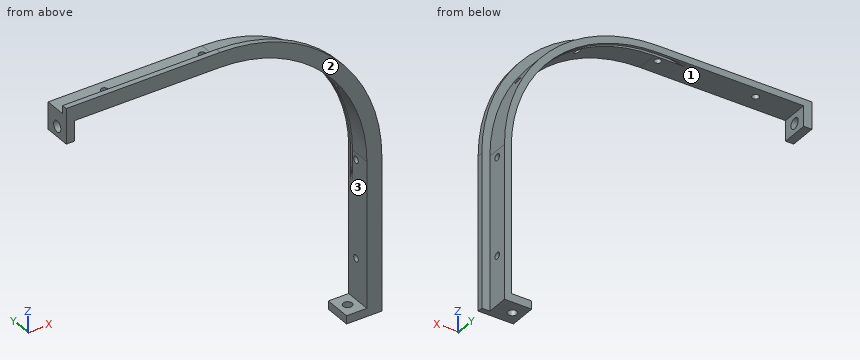
from build123d import *

# Parameters (mm, degrees)
BOSS_EXTRUDE1_DEPTH = 10
CUT_EXTRUDE1_START  = -1
SKETCH2_R           = 55.1
CUT_EXTRUDE1_DEPTH  = 1.1
CUT_EXTRUDE2_DEPTH  = 8
SKETCH4_R           = 2
CUT_EXTRUDE3_DEPTH  = 4
SKETCH5_R           = 1.65
CUT_EXTRUDE4_DEPTH  = 4
SKETCH7_R           = 1.25
CUT_EXTRUDE5_DEPTH  = 114.07
SKETCH9_R           = 1.25
CUT_EXTRUDE6_DEPTH  = 134.776057092


with BuildPart() as part:
    # Sketch1 → Boss-Extrude1 (new body)
    with BuildSketch(Plane(origin=(0, 0, 0), x_dir=(1, 0, 0), z_dir=(0, 1, 0))):
        with BuildLine():
            Line((0, -116.07), (56.57, -116.07))
            ThreePointArc((56.57, -116.07), (98.642853481, -98.642853481), (116.07, -56.57))
            Line((116.07, -56.57), (116.07, 0))
            Line((116.07, 0), (103.07, 0))
            Line((103.07, 0), (103.07, -3))
            Line((103.07, -3), (110.57, -3))
            Line((110.57, -3), (110.57, -56.57))
            ThreePointArc((110.57, -56.57), (94.753766184, -94.753766184), (56.57, -110.57))
            Line((56.57, -110.57), (3, -110.57))
            Line((3, -110.57), (3, -103.07))
            Line((3, -103.07), (0, -103.07))
            Line((0, -103.07), (0, -116.07))
        make_face()
    extrude(amount=BOSS_EXTRUDE1_DEPTH)

    # Sketch2 → Cut-Extrude1 (cut)
    with BuildSketch(Plane(origin=(0, 10, 0), x_dir=(1, 0, 0), z_dir=(0, 1, 0)).offset(CUT_EXTRUDE1_START)):
        with Locations((56.57, -56.57)):
            Circle(SKETCH2_R)
    extrude(amount=-CUT_EXTRUDE1_DEPTH, mode=Mode.SUBTRACT)

    # Sketch3 → Cut-Extrude2 (cut)
    with BuildSketch(Plane(origin=(0, 10, 0), x_dir=(1, 0, 0), z_dir=(0, 1, 0))):
        with BuildLine():
            Line((113.07, -56.57), (113.07, 0))
            Line((113.07, 0), (116.07, 0))
            Line((116.07, 0), (116.07, -56.57))
            ThreePointArc((116.07, -56.57), (98.642853481, -98.642853481), (56.57, -116.07))
            Line((56.57, -116.07), (0, -116.07))
            Line((0, -116.07), (0, -113.07))
            Line((0, -113.07), (56.57, -113.07))
            ThreePointArc((56.57, -113.07), (96.521533137, -96.521533137), (113.07, -56.57))
        make_face()
    extrude(amount=-CUT_EXTRUDE2_DEPTH, mode=Mode.SUBTRACT)

    # Sketch4 → Cut-Extrude3 (cut, through all)
    with BuildSketch(Plane(origin=(3, 0, 0), x_dir=(0, 0, -1), z_dir=(1, 0, 0))):
        with Locations((-106.82, 5)):
            Circle(SKETCH4_R)
    extrude(amount=-CUT_EXTRUDE3_DEPTH, mode=Mode.SUBTRACT)

    # Sketch5 → Cut-Extrude4 (cut, through all)
    with BuildSketch(Plane.XY.offset(3)):
        with Locations((106.82, 5)):
            Circle(SKETCH5_R)
    extrude(amount=-CUT_EXTRUDE4_DEPTH, mode=Mode.SUBTRACT)

    # Sketch7 → Cut-Extrude5 (cut, through all)
    with BuildSketch(Plane.XY.offset(113.07)):
        with Locations((18, 6)):
            Circle(SKETCH7_R)
        with Locations((54, 6)):
            Circle(SKETCH7_R)
    cut_extrude5 = extrude(amount=-CUT_EXTRUDE5_DEPTH, mode=Mode.SUBTRACT)

    # Sketch9 → Cut-Extrude6 (cut, through all)
    with BuildSketch(Plane(origin=(66.888028546, 0, 115.85346386), x_dir=(-0.866025404, 0, 0.5), z_dir=(-0.5, 0, -0.866025404))):
        with Locations((-20.706057092, 6)):
            Circle(SKETCH9_R)
    cut_extrude6 = extrude(amount=CUT_EXTRUDE6_DEPTH, mode=Mode.SUBTRACT)

    # Mirror1: Cut-Extrude5, Cut-Extrude6 across plane
    add(cut_extrude5.mirror(Plane(origin=(0, 0, 0), x_dir=(0.707106781, 0, 0.707106781), z_dir=(-0.707106781, 0, 0.707106781))), mode=Mode.SUBTRACT)
    add(cut_extrude6.mirror(Plane(origin=(0, 0, 0), x_dir=(0.707106781, 0, 0.707106781), z_dir=(-0.707106781, 0, 0.707106781))), mode=Mode.SUBTRACT)


solid = part.part
Geometry: final body of the model. Coordinates: model frame, mm. Face numbers are marked on the shaded views. Round coordinates to 2 decimals unless told otherwise and drop trailing zeros. Loops run counter-clockwise (first coordinate to the right, second up) from the corner with the lowest first, then second, coordinate; pieces in that order, holes last.
Q1. Pin query (flat end, axial travel): P1, Ø3, axis at y = 6, z = 54, coming from the -X side; P2, Ø2.5, axis at y = 5, z = 2, coming from the -X side; P3, Ø6, axis at y = 2.5, z = 108, coming from the +X side. Return the tip coordinate at first contact, or that it passes through.
Q2. Section B-B on z = 91. Return loops of the section in (x, y), plus the area to 3 significant figures.
Q3. Section A-A on x = 29. Return loops of the section in (y, z), plus the area to 3 significant figures.
Q4. Pull-direction query (X, two-part tool) for the marked faces 1, 2 and 3; classes: released by +X, released by -X, zero draft, split by the parting line, or undercut.
Q5. Material intervals for L1, parallel to Y at x = 106.82, z = 2.1; L2, parallel to Y at x = 18, z = 111.75; L3, parallel to X at y = 4, z = 27, sorted ascending.
Q6. Section D-D on z = 34. Return loops of the section in (x, y).
Q7. Section C-C on x = 47. Return loops of the section in (y, z).
Evaluation:
1. P1: stops at x = 110.57
1. P2: stops at x = 103.07
1. P3: stops at x = 91.08
2. outline: (98.17, 0) - (105.1, 0) - (105.1, 2) - (101.37, 2) - (101.37, 10) - (98.17, 10) - (98.17, 9) - (99.59, 9) - (99.59, 7.9) - (98.17, 7.9) - close
2. area: 37.9 mm2
3. outline: (0, 110.57) - (10, 110.57) - (10, 113.07) - (2, 113.07) - (2, 116.07) - (0, 116.07) - close
3. area: 31.0 mm2
4. face 1: undercut
4. face 2: zero draft
4. face 3: released by -X
5. L1: y = 0 to 3.35, 6.65 to 10
5. L2: y = 0 to 4.75, 7.25 to 10
5. L3: x = 110.57 to 113.07
6. outline: (110.57, 0) - (116.07, 0) - (116.07, 2) - (113.07, 2) - (113.07, 10) - (110.57, 10) - close
7. outline: (0, 110.57) - (7.9, 110.57) - (7.9, 110.83) - (9, 110.83) - (9, 110.57) - (10, 110.57) - (10, 113.07) - (2, 113.07) - (2, 116.07) - (0, 116.07) - close
